Verification items for the finished model (mm, model axes). Face numbers are marked on the shaded views. A direction names the side the tool comes from. Round coordinates to 2 decimals unless told otherwise and drop trailing zeros. Write each loop counter-clockwise with the first axis right and the second up, starting at its lowest first coordinate (ties: lowest second). Pieces come first, ordered by that corner, then holes. Notation, with made-up numbers: (12, -13) - (48, -13) arc R23 ccw to (48, 26) - close; hole circle Ø1 at (39, 13). An arc over 180 degrees is marked (long way). Answer as a JSON object with one key per item and string values.
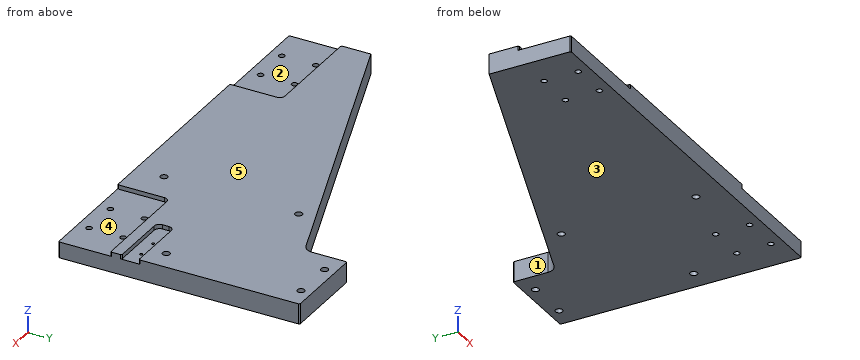
```python
from build123d import *

# Parameters (mm, degrees)
BOSS_EXTRUDE1_DEPTH       = 19.05
CUT_EXTRUDE2_DEPTH        = 4.05
M5_CLEARANCE_HOLE1_D      = 5.5
M5_CLEARANCE_HOLE2_D      = 5.5
M3X0_5_TAPPED_HOLE1_D     = 2.5
M3X0_5_TAPPED_HOLE1_DEPTH = 7.5
M3X0_5_TAPPED_HOLE1_TIP   = 0.751075774
M8X1_25_TAPPED_HOLE1_D    = 6.8
FILLET1_R                 = 10
CHAMFER1_SIZE             = 1


with BuildPart() as part:
    # Sketch1 → Boss-Extrude1 (new body)
    with BuildSketch(Plane.XY):
        Polygon((-195, 50), (-195, -27), (195, -27), (195, 200), (115, 200), (115, 160), align=None)
    extrude(amount=BOSS_EXTRUDE1_DEPTH)

    # Sketch2 → Cut-Extrude2 (cut)
    with BuildSketch(Plane(origin=(0, 0, 0), x_dir=(-1, 0, 0), z_dir=(0, 0, -1))):
        with BuildLine():
            Line((-195, -27), (-95, -27))
            Line((-95, -27), (-95, 17))
            ThreePointArc((-95, 17), (-96.464466094, 20.535533906), (-100, 22))
            Line((-100, 22), (-195, 22))
            Line((-195, 22), (-195, -27))
        make_face()
        with BuildLine():
            Line((195, -27), (195, 22))
            Line((195, 22), (100, 22))
            ThreePointArc((100, 22), (96.464466094, 20.535533906), (95, 17))
            Line((95, 17), (95, -27))
            Line((95, -27), (195, -27))
        make_face()
        with BuildLine():
            Line((-195, 48.5), (-140, 48.5))
            ThreePointArc((-140, 48.5), (-136.464466094, 47.035533906), (-135, 43.5))
            Line((-135, 43.5), (-135, 37.5))
            ThreePointArc((-135, 37.5), (-136.464466094, 33.964466094), (-140, 32.5))
            Line((-140, 32.5), (-195, 32.5))
            Line((-195, 32.5), (-195, 48.5))
        make_face()
    extrude(amount=-CUT_EXTRUDE2_DEPTH, mode=Mode.SUBTRACT)

    # M5 Clearance Hole1 (through all)
    with Locations(Plane(origin=(0, 0, 4.05), x_dir=(-1, 0, 0), z_dir=(0, 0, -1))):
        with Locations((127, 16), (163, 16), (163, -16), (127, -16)):
            Hole(M5_CLEARANCE_HOLE1_D / 2)

    # M5 Clearance Hole2 (through all)
    with Locations(Plane(origin=(0, 0, 4.05), x_dir=(-1, 0, 0), z_dir=(0, 0, -1))):
        with Locations((-163, 16), (-127, 16), (-127, -16), (-163, -16)):
            Hole(M5_CLEARANCE_HOLE2_D / 2)

    # M3x0.5 Tapped Hole1
    with Locations(Plane(origin=(0, 0, 4.05), x_dir=(-1, 0, 0), z_dir=(0, 0, -1))):
        with Locations((-180, 42.5), (-160, 42.5)):
            Hole(M3X0_5_TAPPED_HOLE1_D / 2, depth=M3X0_5_TAPPED_HOLE1_DEPTH)
            with Locations((0, 0, -(M3X0_5_TAPPED_HOLE1_DEPTH + M3X0_5_TAPPED_HOLE1_TIP / 2))):  # 118° drill point
                Cone(0, M3X0_5_TAPPED_HOLE1_D / 2, M3X0_5_TAPPED_HOLE1_TIP, mode=Mode.SUBTRACT)

    # M8x1.25 Tapped Hole1 (through all)
    with Locations(Plane(origin=(0, 0, 0), x_dir=(-1, 0, 0), z_dir=(0, 0, -1))):
        with Locations((-175, 190), (-135, 190), (-65, 126.666666667), (-175, 63.333333333), (-65, 0)):
            Hole(M8X1_25_TAPPED_HOLE1_D / 2)

    # Fillet1
    fillet1_edges = [part.edges().sort_by_distance(p)[0] for p in [
        (115, 160, 9.525),
    ]]
    fillet(fillet1_edges, radius=FILLET1_R)

    # Chamfer1
    chamfer1_edges = [part.edges().sort_by_distance(p)[0] for p in [
        (115, 200, 9.525),
        (195, 200, 9.525),
        (195, -27, 11.55),
        (-195, -27, 11.55),
        (195, 48.5, 2.025),
        (195, 32.5, 2.025),
        (-95, -27, 2.025),
        (-195, 22, 2.025),
        (95, -27, 2.025),
        (195, 22, 2.025),
    ]]
    chamfer(chamfer1_edges, length=CHAMFER1_SIZE)


with BuildPart() as body_2:
    # Mirror1: mirrored copy
    add(part.part.mirror(Plane.XY))


solid = body_2.part
```
1. Go/stop test with flat-tipped pins: pin 1 (2 mm diameter, centred on x = 141, z = -2, fed in from -Y); pin 2 (9 mm diameter, centred on x = 127, y = -16, fed in from +Z); pin 3 (2 mm diameter, centred on y = -8, z = -2, fed in from -X). Record where each tip stops, or that it passes through.
Completed:
{"pin 1": "stops at y = 22", "pin 2": "stops at z = -4.05", "pin 3": "stops at x = -95"}
2. Material ranges on probe 1 along Y at (x, z) = (175, -9); probe 2 along Y at (x, z) = (127, -14); probe 3 along Y at (x, z) = (135, -5), recorded low to high. Write a range as from..to.
Completed:
{"probe 1": "y = -27..59.93, 66.73..186.6, 193.4..200", "probe 2": "y = -27..-18.75, -13.25..13.25, 18.75..200", "probe 3": "y = -27..186.6, 193.4..200"}
3. Cross-section at A-A (z = -7). Count the separate pieces of the cut face and the enclosed holes in it, plus the area to 3 significant figures.
Completed:
{"separate pieces": "1", "enclosed holes": "15", "area": "58,700 mm^2"}
4. Cross-section at B-B (y = 100). Record the boundary of the cut face in (x, z).
Completed:
{"outline": "(-54.09, -19.05) - (195, -19.05) - (195, 0) - (-54.09, 0) - close"}
5. Cross-section at C-C (x = -63.5). Record the boundary of the cut face in (y, z), plus the area to 3 significant figures.
Completed:
{"outline": "(-27, -19.05) - (96.66, -19.05) - (96.66, 0) - (-27, 0) - close", "area": "2,360 mm^2"}
6. Access from +Z, -Z, +X, -X, +Y, -Y to the whole of each face (thin tool, end or side, straight path). Record for the marked faces 1, 2, 3, 4 and 5.
Completed:
{"face 1": "+Z, -Z, -X, +Y", "face 2": "+Z, -X, -Y", "face 3": "-Z, +X, -X, +Y, -Y", "face 4": "+Z, +X, -Y", "face 5": "+Z, +X, -X, +Y, -Y"}
